Job drawing, mm, ordinate dimensions from the low corner. One solid piece. A direction names the side the tool comes from. Give positions to 0.01 mm unless a question says otherwise; leave off trailing zeros. Order: outer loops, then holes, each group sorted by start corner. A loop starts at its lowest first (then second) coordinate and runs counter-clockwise, first axis right, second up. Notation, with made-up numbers: (-6.75, 26.25) -> (24.25, 26.25) arc R19 ccw to (24.25, 57.25) -> close; hole circle Ø4 at (67, 25). An arc over 180 degrees is marked (long way). Write item = value, one per line. Start each with the question number.
(1) Saw through at B-B, the plane z = 66. List the corners of the cut face in (x, y), then the cut area to 3 significant figures.
(2) Probe line 1 along X through (y, z) = (31.5, 25); line 2 along Z through (x, y) = (111.75, 40); line 3 along Y through (x, z) = (60, 112). List the from-to ranges inside material, lowest first. Write a range as from..to.
(3) Flat gauge pins, fed straight in: pin 1 (3 mm diameter, centred on x = 90.5, y = 59, fed in from -Z); pin 2 (18 mm diameter, centred on x = 76, y = 28, fed in from +Z). Where does each tip first touch, or does it go through?
(4) Saw through at C-C, the plane x = 14. List the corners of the cut face in (y, z).
(5) Two-plate mould, pull along Z, no slides. Class the marked faces 6, 7, 8 and 9: pulls with the +Z half, pulls with the -Z half, needs draft (parallel to the pull), parting line crosses it, or undercut.
(6) Saw through at D-D, the plane z = 36. List the corners of the cut face in (x, y), then the cut area to 3 significant figures.
(7) Which spindle directions (+Z, -Z, +X, -X, +Y, -Y) get a long thin tool onto all of the face, cutting with end or side? Do the marked faces 1, 2, 3, 4 and 5. Say none if no direction does.
(8) Saw through at A-A, the plane y = 40. List the corners of the cut face in (x, z), then the cut area to 3 significant figures.
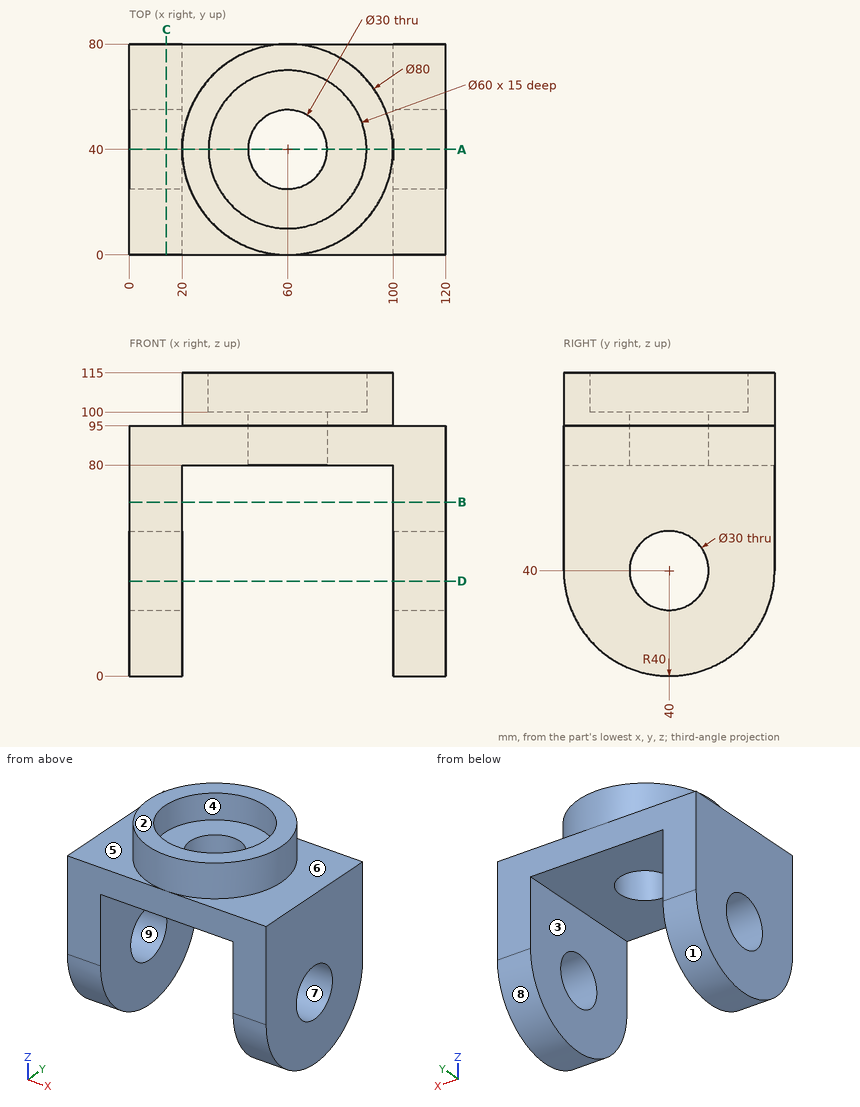
Results list:
q1.outline = (0, 0) -> (20, 0) -> (20, 80) -> (0, 80) -> close; (100, 0) -> (120, 0) -> (120, 80) -> (100, 80) -> close
q1.area = 3,200 mm^2
q2.line_1 = 0..20, 100..120
q2.line_2 = 0..25, 55..95
q2.line_3 = 0..10, 70..80
q3.pin_1 = 80
q3.pin_2 = 100
q4.outline = (0, 40) arc R40 ccw to (80, 40) -> (80, 95) -> (0, 95) -> close; hole circle Ø30 at (40, 40)
q5.face_6 = pulls with the +Z half
q5.face_7 = undercut
q5.face_8 = pulls with the -Z half
q5.face_9 = undercut
q6.outline = (0, 0.2) -> (20, 0.2) -> (20, 25.54) -> (0, 25.54) -> close; (0, 54.46) -> (20, 54.46) -> (20, 79.8) -> (0, 79.8) -> close; (100, 0.2) -> (120, 0.2) -> (120, 25.54) -> (100, 25.54) -> close; (100, 54.46) -> (120, 54.46) -> (120, 79.8) -> (100, 79.8) -> close
q6.area = 2,030 mm^2
q7.face_1 = -Z, +X, -X
q7.face_2 = +Z, +X, -X, +Y, -Y
q7.face_3 = -Z, +Y, -Y
q7.face_4 = +Z
q7.face_5 = +Z, -X
q8.outline = (0, 0) -> (20, 0) -> (20, 25) -> (0, 25) -> close; (0, 55) -> (20, 55) -> (20, 80) -> (45, 80) -> (45, 100) -> (30, 100) -> (30, 115) -> (20, 115) -> (20, 95) -> (0, 95) -> close; (75, 80) -> (100, 80) -> (100, 55) -> (120, 55) -> (120, 95) -> (100, 95) -> (100, 115) -> (90, 115) -> (90, 100) -> (75, 100) -> close; (100, 0) -> (120, 0) -> (120, 25) -> (100, 25) -> close
q8.area = 3,900 mm^2
